The drawing under review shows one solid part. Ordinate dimensions are in mm from its lowest x, y, z. A direction names the side the tool comes from. Give positions to 0.01 mm unless a question says otherwise; leave off trailing zeros. Loops run counter-clockwise (first coordinate to the right, second up) from the corner with the lowest first, then second, coordinate; pieces in that order, holes last. Notation, with made-up numbers: M -25.75,62 L -8.75,62 A21 cw -8.75,88 Z; hole C 27.5,-18.75 d7. An arc over 180 degrees is marked long. Put each result on its own line as item: value. Start each with the question number.
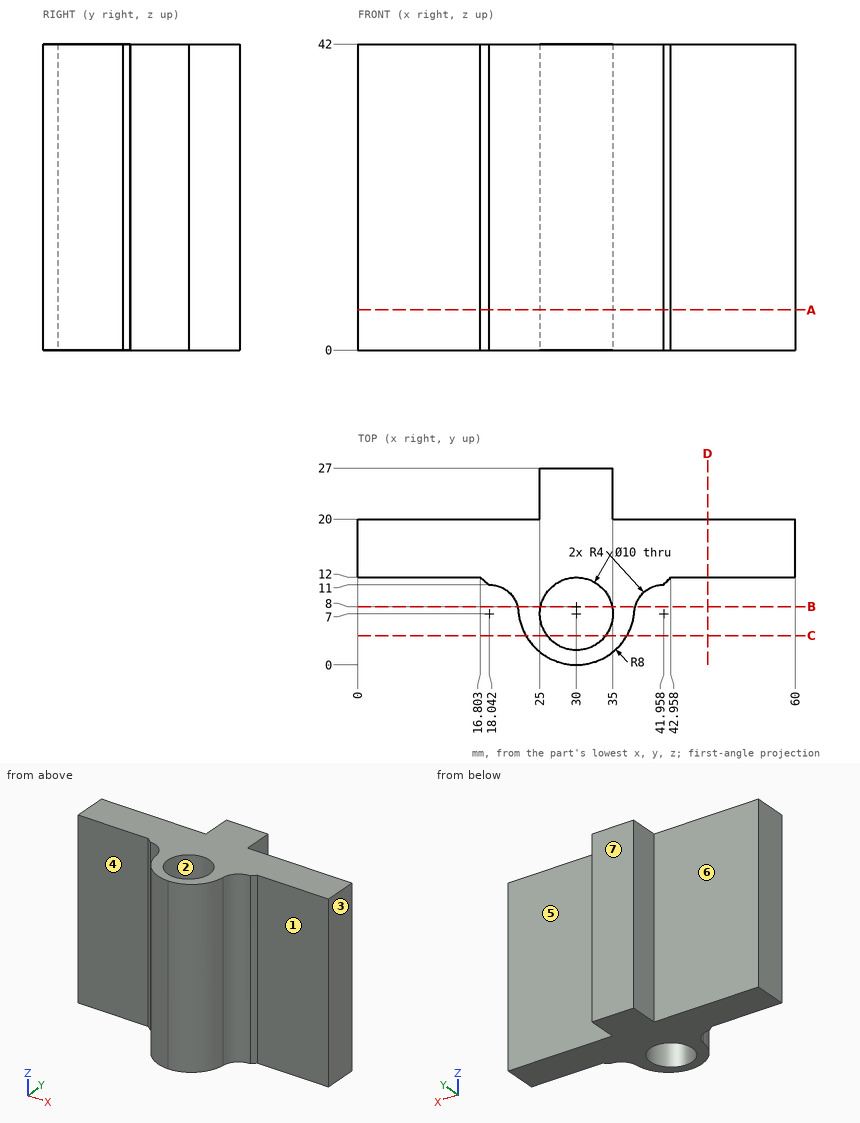
Item 1: To check wall thickness, follow L1, parallel to Y at x = 30, z = 17; L2, parallel to Y at x = 25.5, z = 40 (1 decimal); L3, parallel to Y at x = 45, z = 36. State the ranges of each line that lie inside material, in increasing order. Write a range as [from, to].
Item 2: Tool access review of the marked faces 4, 5, 6 and 7: name each direction out of +Z, -Z, +X, -X, +Y, -Y from which nothing blocks a thin tool from reaching the whole face with its end or side.
Item 3: Draft analysis for pull direction Y (two halves, no side actions). For the marked faces 1, 2 and 3, state which applies: +Y half, -Y half, draft (parallel to the pull), parting line (faces both ways), or undercut.
Item 4: Consider section D-D, the plane x = 48. Write out the cut boundary in (y, z), plus the area to 3 significant figures.
Item 5: Consider section C-C, the plane y = 4. Write out the cut boundary in (x, z), plus the area to 3 significant figures.
Item 6: Clearance check with flat-ended pins moving along their axes: pin 1 Ø1.5 at (x, z) = (47, 6) entering from -Y; pin 2 Ø2 at (y, z) = (24.5, 25.5) entering from +X; pin 3 Ø3 at (x, z) = (25, 32.5) entering from -Y; pin 4 Ø6 at (y, z) = (15.5, 16) entering from -X. State where each tip first meets the part, or that it passes through.
Item 7: Consider section A-A, the plane z = 5.5. Write out the cut boundary in (x, y).
Item 8: Consider section B-B, the plane y = 8. Write out the cut boundary in (x, z) (1 decimal), plus the area to 3 significant figures.
Report:
1. L1: [0, 2], [12, 27]
1. L2: [1.4, 4.8], [9.2, 27]
1. L3: [12, 20]
2. face 4: +Z, -Z, -X, -Y
2. face 5: +Z, -Z, +X, +Y
2. face 6: +Z, -Z, -X, +Y
2. face 7: +Z, -Z, +X, -X, +Y
3. face 1: -Y half
3. face 2: undercut
3. face 3: draft
4. outline: M 12,0 L 20,0 L 20,42 L 12,42 Z
4. area: 336 mm²
5. outline: M 23.07,0 L 26,0 L 26,42 L 23.07,42 Z; M 34,0 L 36.93,0 L 36.93,42 L 34,42 Z
5. area: 246 mm²
6. pin 1: y = 12
6. pin 2: x = 35
6. pin 3: y = 0.81
6. pin 4: x = 0
7. outline: M 0,12 L 16.8,12 L 18.04,11 A4 cw 22.03,7.33 A8 ccw 37.97,7.33 A4 cw 41.96,11 L 42.96,12 L 60,12 L 60,20 L 35,20 L 35,27 L 25,27 L 25,20 L 0,20 Z; hole C 30,7 d10
8. outline: M 21.9,0 L 25.1,0 L 25.1,42 L 21.9,42 Z; M 34.9,0 L 38.1,0 L 38.1,42 L 34.9,42 Z
8. area: 268 mm²
